Geometry check sheet. Reference: the model listing, model coordinates, mm. A direction names the side the tool comes from. Coordinates: 2 decimals unless noted, no trailing zeros. Write each loop counter-clockwise with the first axis right and the second up, starting at its lowest first coordinate (ties: lowest second). Pieces come first, ordered by that corner, then holes. Notation, with made-up numbers: (63, 65.25) -> (83, 65.25) arc R28 cw to (83, 92.25) -> close; hole circle Ø2 at (29.5, 39.25). An arc over 180 degrees is marked (long way). Use a Markdown table: item, result.
Autodesk Inventor part; units mm, degrees
ref_plane "YZ Plane" through (0, 0, 0) normal (1, 0, 0) x (0, 1, 0)
ref_plane "XZ Plane" through (0, 0, 0) normal (0, 1, 0) x (-1, 0, 0)
ref_plane "XY Plane" through (0, 0, 0) normal (0, 0, 1) x (1, 0, 0)
sketch "스케치4" plane through (0, 0, 0) normal (0, 1, 0) x (-1, 0, 0)
  line L0 (0, 0) -> (-12, 0)
  line L1 (-12, 0) -> (-12, -4.5)
  line L2 (-12, -4.5) -> (0, -4.5)
  line L3 (0, -4.5) -> (0, 0)
  dimension "d18" = 12
  dimension "d19" = 4.5
extrude "돌출5" add sketch "스케치4" along normal blind 6
sketch "스케치5" plane through (0, 6, 0) normal (0, 1, 0) x (1, 0, 0)
  line L0 (12, 0) -> (12, 4.5)
  line L1 (12, 2.25) -> (12, 3.25)
  line L2 (12, 3.25) -> (6.5, 3.25)
  line L3 (6.5, 3.25) -> (8.5, 3.25)
  line L4 (8.5, 3.25) -> (8.5, 1.25)
  line L5 (8.5, 1.25) -> (6.5, 1.25)
  line L6 (6.5, 1.25) -> (6.5, 3.25)
  point P0 (0, 0)
  dimension "d22" = 1
  dimension "d23" = 5.5
  dimension "d24" = 2
  dimension "d25" = 2
extrude "돌출6" add sketch "스케치5" along normal blind 4
sketch "스케치6" plane through (0, 0, 0) normal (0, -1, 0) x (1, 0, 0)
  line L0 (0, 0) -> (12, 0)
  line L1 (6, 0) -> (6, -2.25)
  line L2 (6, -2.25) -> (9, -2.25)
  line L3 (9, -2.25) -> (3, -2.25)
  circle A0 centre (6, -2.25) radius 0.375
  circle A1 centre (9, -2.25) radius 0.375
  circle A2 centre (3, -2.25) radius 0.375
  dimension "d28" = 2.25
  dimension "d29" = 3
  dimension "d30" = 6
  dimension "d31" = 0.75
  dimension "d32" = 0.75
  dimension "d33" = 0.75
extrude "돌출7" add sketch "스케치6" along normal blind 3
properties part number "tmdnlcl"
Item 1: Tool access check on faces 1 (the flat face through (6.5, 8, -2)), 2 (the flat face through (8, 8, -1.25)), 3 (the flat face through (8, 8, -3.25)). Record the directions out of +Z, -Z, +X, -X, +Y, -Y that give a thin tool (end or side, any length) a straight path to the whole face; none if there is none.
Answer block:
| item | result |
|---|---|
| face 1 | +Z, -Z, -X, +Y |
| face 2 | +Z, +X, -X, +Y |
| face 3 | -Z, +X, -X, +Y |
Item 2: Section check D-D on y = 7.25. Record the boundary of the cut face in (x, z), then the cut area to 3 significant figures.
Answer block:
| item | result |
|---|---|
| outline | (6.5, -3.25) -> (8.5, -3.25) -> (8.5, -1.25) -> (6.5, -1.25) -> close |
| area | 4.00 mm^2 |
Item 3: Section check C-C on z = -1.45. Record the boundary of the cut face in (x, y).
Answer block:
| item | result |
|---|---|
| outline | (0, 0) -> (12, 0) -> (12, 6) -> (8.5, 6) -> (8.5, 10) -> (6.5, 10) -> (6.5, 6) -> (0, 6) -> close |
Item 4: Section check A-A on x = 7. Record the boundary of the cut face in (y, z), then the cut area to 3 significant figures.
Answer block:
| item | result |
|---|---|
| outline | (0, -4.5) -> (6, -4.5) -> (6, -3.25) -> (10, -3.25) -> (10, -1.25) -> (6, -1.25) -> (6, 0) -> (0, 0) -> close |
| area | 35.0 mm^2 |
Item 5: Section check B-B on z = -2.25. Record the boundary of the cut face in (x, y) (3 decimals), then the cut area to 4 significant figures.
Answer block:
| item | result |
|---|---|
| outline | (0, 0) -> (2.625, 0) -> (2.625, -3) -> (3.375, -3) -> (3.375, 0) -> (5.625, 0) -> (5.625, -3) -> (6.375, -3) -> (6.375, 0) -> (8.625, 0) -> (8.625, -3) -> (9.375, -3) -> (9.375, 0) -> (12, 0) -> (12, 6) -> (8.5, 6) -> (8.5, 10) -> (6.5, 10) -> (6.5, 6) -> (0, 6) -> close |
| area | 86.75 mm^2 |
Item 6: Thickness scan on L1, parallel to Y at x = 9.5, z = -2.5; L2, parallel to X at y = 7.25, z = -2.8; L3, parallel to Z at x = 8, y = 7.25. Record the ranges inside material, lowest first. Write a range as [from, to].
Answer block:
| item | result |
|---|---|
| L1 | y = [0, 6] |
| L2 | x = [6.5, 8.5] |
| L3 | z = [-3.25, -1.25] |
Item 7: Depth check by flat-ended pin: P1, Ø1.6, axis at y = 7, z = -2.5, coming from the -X side; P2, Ø2, axis at x = 7.5, y = 8, coming from the +Z side; P3, Ø1, axis at x = 7, y = 7, coming from the -Z side. Enter the tip coordinate at first touch or a pass-through.
Answer block:
| item | result |
|---|---|
| P1 | stops at x = 6.5 |
| P2 | stops at z = -1.25 |
| P3 | stops at z = -3.25 |
